Work out the finished part from the listing and answer in its coordinate system (mm). A direction names the side the tool comes from. Round coordinates to 2 decimals unless told otherwise and drop trailing zeros. Write each loop counter-clockwise with the first axis right and the second up, starting at its lowest first coordinate (ties: lowest second). Pieces come first, ordered by that corner, then holes. Notation, with made-up numbers: M -34.75,3.5 L 18.25,3.5 A10 cw 18.25,11.5 Z; hole C 79.25,24.25 d6. An arc over 180 degrees is marked long. One line per item, written item: value. Start each with the question number.
Q1. Find section D-D (x = 12). Write down the section's boundary in (y, z).
Q2. Find section C-C (z = -25). Write down the section's boundary in (x, y).
Q3. Consider probe 1 along Y at (x, z) = (6.5, -3.8); probe 2 along X at (y, z) = (36.7, -25); probe 3 along Y at (x, z) = (5, -21). Determine where each line is inside the solid, lowest interval first.
Q4. A tool of negligible diameter and unlimited length cuts with its end or side. For faces 5 (the flat face through (4, 18, -5)), 6 (the cylindrical face through (7.87, 36.67, -27.15)), from which of +Z, -Z, +X, -X, +Y, -Y can it reach the whole face along a straight path? Write none if from no direction.
Q5. Find section A-A (y = 18.7). Write down the section's boundary in (x, z), and give its area (3 significant figures).
Q6. The mould has two halves that part along X. Classify faces 1 (the cylindrical face through (6.721, 20.386, -2.535)), 2 (the flat face through (0, 24.9, -4.6)), 3 (the flat face through (13, 24.9, -4.6)), 4 (the flat face through (6, 0, -3)): released by +X, released by -X, zero draft, split by the parting line, or undercut.
Q7. Find section B-B (x = 6.5). Write down the section's boundary in (y, z), and give its area (3 significant figures).
Q8. Given pin 1 Ø2.5 at (x, y) = (6.5, 4) entering from +Z; pin 2 Ø4 at (x, z) = (9.5, -27) entering from -Y; pin 3 Ø4 at (x, y) = (6.5, 18.7) entering from -Z, each flat-ended and moving along its own axis, determine where each tip first touches the part or whether it passes through.
from build123d import *

# Parameters (mm, degrees)
BOSS_EXTRUDE1_DEPTH = 13
SKETCH2_R           = 1.7
CUT_EXTRUDE1_DEPTH  = 6
SKETCH3_R           = 2.55
CUT_EXTRUDE2_DEPTH  = 39.3


with BuildPart() as part:
    # Sketch1 → Boss-Extrude1 (new body)
    with BuildSketch(Plane(origin=(0, 0, 0), x_dir=(0, 0, -1), z_dir=(1, 0, 0))):
        Polygon((0, 0), (0, 38.3), (35, 38.3), (35, 35), (5, 35), (5, 0), align=None)
    extrude(amount=BOSS_EXTRUDE1_DEPTH)

    # Sketch2 → Cut-Extrude1 (cut, through all)
    with BuildSketch(Plane(origin=(0, 0, -5), x_dir=(-1, 0, 0), z_dir=(0, 0, -1))):
        with Locations((-6.5, 18.7)):
            Circle(SKETCH2_R)
        with Locations((-6.5, 4)):
            Circle(SKETCH2_R)
    extrude(amount=-CUT_EXTRUDE1_DEPTH, mode=Mode.SUBTRACT)

    # Sketch3 → Cut-Extrude2 (cut, through all)
    with BuildSketch(Plane(origin=(0, 38.3, 0), x_dir=(1, 0, 0), z_dir=(0, 1, 0))):
        with Locations((6.5, 25)):
            Circle(SKETCH3_R)
    extrude(amount=-CUT_EXTRUDE2_DEPTH, mode=Mode.SUBTRACT)


solid = part.part
The answers:
1. outline: M 0,-5 L 35,-5 L 35,-35 L 38.3,-35 L 38.3,0 L 0,0 Z
2. outline: M 0,35 L 3.95,35 L 3.95,38.3 L 0,38.3 Z; M 9.05,35 L 13,35 L 13,38.3 L 9.05,38.3 Z
3. probe 1: 0 to 2.3, 5.7 to 17, 20.4 to 38.3
3. probe 2: 0 to 3.95, 9.05 to 13
3. probe 3: 35 to 38.3
4. face 5: -Z, +X, -X, -Y
4. face 6: +Y, -Y
5. outline: M 0,-5 L 4.8,-5 L 4.8,0 L 0,0 Z; M 8.2,-5 L 13,-5 L 13,0 L 8.2,0 Z
5. area: 48.0 mm2
6. face 1: undercut
6. face 2: released by -X
6. face 3: released by +X
6. face 4: zero draft
7. outline: M 0,-5 L 2.3,-5 L 2.3,0 L 0,0 Z; M 5.7,-5 L 17,-5 L 17,0 L 5.7,0 Z; M 20.4,-5 L 35,-5 L 35,-22.45 L 38.3,-22.45 L 38.3,0 L 20.4,0 Z; M 35,-35 L 38.3,-35 L 38.3,-27.55 L 35,-27.55 Z
7. area: 240 mm2
8. pin 1: through
8. pin 2: y = 35
8. pin 3: z = -5
